from build123d import *

# Parameters (mm, degrees)
SKETCH1_W           = 6
SKETCH1_H           = 6
SKETCH1_R           = 1.75
BOSS_EXTRUDE1_DEPTH = 3
SKETCH2_W           = 6
SKETCH2_H           = 6
BOSS_EXTRUDE2_DEPTH = 1.5
SKETCH3_R           = 0.2
BOSS_EXTRUDE3_DEPTH = 3.8


with BuildPart() as part:
    # Sketch1 → Boss-Extrude1 (new body)
    with BuildSketch(Plane.XY):
        with Locations((3, 3)):
            Rectangle(SKETCH1_W, SKETCH1_H)
        with Locations((3, 3)):
            Circle(SKETCH1_R, mode=Mode.SUBTRACT)
    extrude(amount=BOSS_EXTRUDE1_DEPTH)

    # Sketch2 → Boss-Extrude2 (add)
    with BuildSketch(Plane.XY):
        with Locations((3, 3)):
            Rectangle(SKETCH2_W, SKETCH2_H)
    extrude(amount=BOSS_EXTRUDE2_DEPTH)

    # Sketch3 → Boss-Extrude3 (add)
    with BuildSketch(Plane.XZ):
        with Locations(Location((1.2, 0.5, 0), (0, 0, 90))):
            Circle(SKETCH3_R)
        with Locations(Location((4.8, 0.5, 0), (0, 0, 90))):
            Circle(SKETCH3_R)
    extrude(amount=BOSS_EXTRUDE3_DEPTH)


solid = part.part
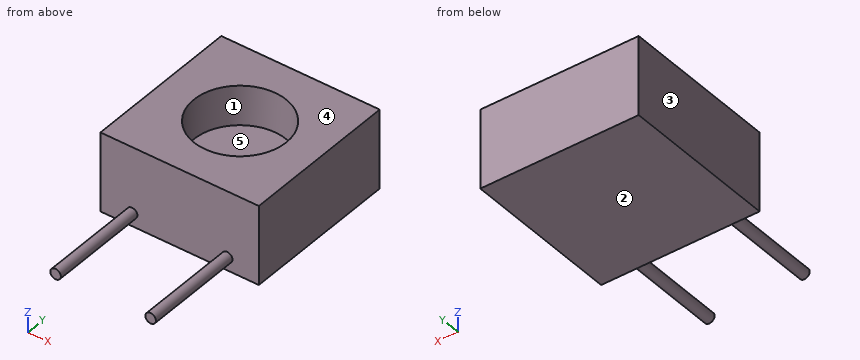
Geometry check sheet. Reference: the model listing, model coordinates, mm. Face numbers are marked on the shaded views. A direction names the side the tool comes from. Give positions to 0.01 mm unless a question says otherwise; leave off trailing zeros. Write each loop counter-clockwise with the first axis right and the second up, starting at its lowest first coordinate (ties: lowest second). Pieces come first, ordered by that corner, then holes. Notation, with made-up numbers: (31.5, 85) - (68.5, 85) arc R36 cw to (68.5, 124) - close; hole circle Ø10 at (21.5, 35.5). An arc over 180 degrees is marked (long way). Put each result on its own line as item: value.
1. Sectioned sample at B-B, the plane y = -2. Enter the section's corners in (x, z), plus the area to 3 significant figures.
Ans:
outline: circle Ø0.4 at (1.2, 0.5); circle Ø0.4 at (4.8, 0.5)
area: 0.251 mm²
2. Sectioned sample at C-C, the plane x = 3. Enter the section's corners in (y, z).
Ans:
outline: (0, 0) - (6, 0) - (6, 3) - (4.75, 3) - (4.75, 1.5) - (1.25, 1.5) - (1.25, 3) - (0, 3) - close
3. Draft check along X on the marked faces 1, 2 and 3. Enter one of: +X half, -X half, draft (parallel to the pull), parting line (faces both ways), or undercut.
Ans:
face 1: undercut
face 2: draft
face 3: -X half
4. Sectioned sample at A-A, the plane z = 1.9. Enter the section's corners in (x, y), plus the area to 3 significant figures.
Ans:
outline: (0, 0) - (6, 0) - (6, 6) - (0, 6) - close; hole circle Ø3.5 at (3, 3)
area: 26.4 mm²
5. Set-up check for the marked faces 4 and 5: record each of +Z, -Z, +X, -X, +Y, -Y from which the full face is reachable in a straight line by a thin tool's end or side.
Ans:
face 4: +Z, +X, -X, +Y, -Y
face 5: +Z
6. Go/stop test with flat-tipped pins: pin 1 (1 mm diameter, centred on y = -1, z = 1.5, fed in from +X); pin 2 (3 mm diameter, centred on x = 3, y = 3, fed in from +Z); pin 3 (1.5 mm diameter, centred on x = 2.5, z = 2, fed in from -Y). Record where each tip stops, or that it passes through.
Ans:
pin 1: passes through
pin 2: stops at z = 1.5
pin 3: stops at y = 0
7. Thickness scan on line 1 (Y direction, x = 3, z = 2); line 2 (Y direction, x = 2.65, z = 1). Record the ranges inside material, lowest first.
Ans:
line 1: y = 0 to 1.25, 4.75 to 6
line 2: y = 0 to 6
